from build123d import *

# Parameters (mm, degrees)
SKETCH1_R           = 1.5
BOSS_EXTRUDE1_DEPTH = 4
FILLET1_R           = 1


with BuildPart() as part:
    # Sketch1 → Boss-Extrude1 (new body)
    with BuildSketch(Plane(origin=(0, 0, 0), x_dir=(0, 0, -1), z_dir=(1, 0, 0))):
        with BuildLine():
            Line((2, -3.464101615), (23.015290845, 8.669082211))
            ThreePointArc((23.015290845, 8.669082211), (25.733387782, 9.3341963), (28.383173027, 8.434715414))
            Line((28.383173027, 8.434715414), (51.232670073, -7.564674663))
            Line((51.232670073, -7.564674663), (56.023067, -8.799461594))
            Line((56.023067, -8.799461594), (57.638075063, -7.307602004))
            Line((57.638075063, -7.307602004), (58.156839412, -9.349469104))
            Line((58.156839412, -9.349469104), (59.53422498, -8.07711269))
            Line((59.53422498, -8.07711269), (59.976661488, -9.818551844))
            Line((59.976661488, -9.818551844), (61.239859239, -8.642065932))
            Line((61.239859239, -8.642065932), (61.648229646, -10.249420215))
            Line((61.648229646, -10.249420215), (62.934954569, -9.051022147))
            Line((62.934954569, -9.051022147), (63.350930911, -10.688313547))
            Line((63.350930911, -10.688313547), (64.567456775, -9.58151124))
            Line((64.567456775, -9.58151124), (65.081008751, -11.134263546))
            Line((65.081008751, -11.134263546), (68.163696398, -11.928866264))
            Line((68.163696398, -11.928866264), (69.232670073, -10.40221364))
            Line((69.232670073, -10.40221364), (28.796925265, 17.911199687))
            ThreePointArc((28.796925265, 17.911199687), (26.147140021, 18.810680574), (23.429043084, 18.145566485))
            Line((23.429043084, 18.145566485), (-2, 3.464101615))
            ThreePointArc((-2, 3.464101615), (-3.464101615, -2), (2, -3.464101615))
        make_face()
        Circle(SKETCH1_R, mode=Mode.SUBTRACT)
        with Locations((25.980762114, 15)):
            Circle(SKETCH1_R, mode=Mode.SUBTRACT)
    extrude(amount=BOSS_EXTRUDE1_DEPTH)

    # Fillet1
    fillet1_edges = [part.edges().sort_by_distance(p)[0] for p in [
        (4, 9.3341963, -25.733387782),
        (4, 0.435020376, -39.80792155),
        (0, 10.80483405, -10.714521542),
        (0, 18.810680574, -26.147140021),
        (0, 3.754493023, -49.014797669),
        (0, 0.435020376, -39.80792155),
        (0, 9.3341963, -25.733387782),
        (0, 2.602490298, -12.507645422),
        (0, -2, 3.464101615),
        (4, -2, 3.464101615),
        (4, 3.754493023, -49.014797669),
        (4, 18.810680574, -26.147140021),
        (4, 10.80483405, -10.714521542),
        (4, 2.602490298, -12.507645422),
    ]]
    fillet(fillet1_edges, radius=FILLET1_R)


solid = part.part
Check sheet for the modelled part. Datum: model origin and axes. Units: mm. A direction names the side the tool comes from. Give positions to 0.01 mm unless a question says otherwise; leave off trailing zeros. Answer as a JSON object with one key per item and string values. Group by question number.
Q1. Access from +Z, -Z, +X, -X, +Y, -Y to the whole of each face (thin tool, end or side, straight path). Record for faces 1 (the cylindrical face through (3.699, 10.455, -10.679)), 2 (the flat face through (1.986, 2.518, -12.361)), 3 (the cylindrical face through (0.301, 2.934, -12.512)).
Q2. Release check for a two-part mould opening along Z. For faces 4 (the flat face through (1.972, -8.173, -53.594)), 5 (the flat face through (0, 7, -33)), 6 (the cylindrical face through (1.97, 15.45, -27.41)), 7 (the cylindrical face through (1.99, 18.81, -26.19)) record: released by +Z, released by -Z, zero draft, split by the parting line, or undercut.
Q3. Material ranges on line 1 along Z through (x, y) = (1.8, 14); line 2 along Z through (x, y) = (1.9, 3); line 3 along Y through (x, z) = (1.7, 0), recorded low to high. Write a range as [from, to].
Q4. Cross-section at A-A on y = 0. Give the number of separate pieces and of enclosed holes in the cut face, then the cut area to 3 significant figures.
Q5. Go/stop test with flat-tipped pins: P1, Ø1.5, axis at x = 3.5, z = -16, coming from the +Y side; P2, Ø1.5, axis at x = 3, z = -33.5, coming from the -Y side. Record where each tip stops, or that it passes through.
Evaluation:
{
 "1": {"face 1": "+Z, +X, +Y", "face 2": "+X, -X, -Y", "face 3": "-X, -Y"},
 "2": {"face 4": "released by +Z", "face 5": "zero draft", "face 6": "undercut", "face 7": "split by the parting line"},
 "3": {"line 1": "z = [-34.38, -27.1], [-24.86, -16.25]", "line 2": "z = [-50.09, -36.14], [-13.2, 2.65]", "line 3": "y = [-4, -1.5], [1.5, 4.62]"},
 "4": {"separate pieces": "3", "enclosed holes": "0", "area": "89.0 mm2"},
 "5": {"P1": "stops at y = 14.23", "P2": "stops at y = 4.33"}
}
